Autodesk Inventor part; units mm, degrees
ref_plane "YZ Plane" through (0, 0, 0) normal (1, 0, 0) x (0, 1, 0)
ref_plane "XZ Plane" through (0, 0, 0) normal (0, 1, 0) x (-1, 0, 0)
ref_plane "XY Plane" through (0, 0, 0) normal (0, 0, 1) x (1, 0, 0)
sketch "スケッチ2" plane through (0, 0, 0) normal (0, 1, 0) x (-1, 0, 0)
  line L0 (43, -215) -> (-441.4, 962.3333)
  line L1 (32, 0) -> (32, -200)
  line L2 (0, 0) -> (0, -200)
  line L3 (32, 0) -> (0, 0)
  line L4 (16, 0) -> (16, -149.3765)
  line L5 (32, -200) -> (0, -200)
  dimension "d0" = 50.6234
ref_plane "作業平面1" through (-32, 0, -200) normal (0, 0, 1) x (1, 0, 0)
sketch "スケッチ5" plane through (-32, 0, -200) normal (0, 0, 1) x (1, 0, 0)
  line L0 (0, -16) -> (32, -16)
  line L1 (32, -16) -> (32, 16)
  line L2 (32, 16) -> (0, 16)
  line L3 (0, 16) -> (0, -16)
  line L4 (0, -16) -> (32, 16) construction
  line L5 (32, -16) -> (0, 16) construction
  line L6 (29.7, -13.7) -> (2.3, -13.7)
  line L7 (2.3, -13.7) -> (2.3, 13.7)
  line L8 (2.3, 13.7) -> (29.7, 13.7)
  line L9 (29.7, 13.7) -> (29.7, -13.7)
  point P0 (32, 0)
  point P1 (16, 0)
  dimension "d7" = 32
  dimension "d8" = 32
  dimension "d9" = 2.3
extrude "押し出し2" add sketch "スケッチ5" along normal blind 70
sketch "スケッチ6" plane through (-32, -16, -200) normal (0, -1, 0) x (1, 0, 0)
  line L0 (-11, -15) -> (473.4, 1162.3333)
  line L1 (16, 200) -> (16, 50.6235)
  point P0 (32, 200)
hole "穴1" at (-16, -16, -149.3765) direction (0, 1, 0) diameter 10 end through all
properties part number "ステア棒"
Read the model definition and answer for the solid it produces. Units are mm, in the model's axes. A direction names the side the tool comes from. Coordinates: 2 decimals unless noted, no trailing zeros. Write each loop counter-clockwise with the first axis right and the second up, starting at its lowest first coordinate (ties: lowest second). Pieces come first, ordered by that corner, then holes. Notation, with made-up numbers: (67.25, 41) - (75.25, 41) arc R27 ccw to (75.25, 73) - close; hole circle Ø5 at (10, 37.25). An arc over 180 degrees is marked (long way). One line per question, with ' | ' between items.
Q1. Find section B-B, the plane y = -3. Write down the section's boundary in (x, z), plus the area to 3 significant figures.
Result set:
outline: (-32, -200) - (-29.7, -200) - (-29.7, -130) - (-32, -130) - close; (-2.3, -200) - (0, -200) - (0, -130) - (-2.3, -130) - close | area: 322 mm^2
Q2. Find section A-A, the plane x = -6. Write down the section's boundary in (y, z), plus the area to 3 significant figures.
Result set:
outline: (-16, -200) - (-13.7, -200) - (-13.7, -130) - (-16, -130) - close; (13.7, -200) - (16, -200) - (16, -130) - (13.7, -130) - close | area: 322 mm^2
Q3. Find section C-C, the plane z = -141.5. Write down the section's boundary in (x, y), plus the area to 3 significant figures.
Result set:
outline: (-32, -16) - (0, -16) - (0, 16) - (-32, 16) - close; hole (-29.7, -13.7) - (-2.3, -13.7) - (-2.3, 13.7) - (-29.7, 13.7) - close | area: 273 mm^2
Q4. Determine the mould class of faces 3 (the cylindrical face through (-17.502, 14.866, -154.146)), 4 (the flat face through (-32, 0, -165)), 5 (the flat face through (-2, 0, -200)) for opening direction Z: +Z half, -Z half, draft (parallel to the pull), parting line (faces both ways), or undercut.
Result set:
face 3: undercut | face 4: draft | face 5: -Z half
Q5. Find section D-D, the plane x = -16. Write down the section's boundary in (y, z), plus the area to 3 significant figures.
Result set:
outline: (-16, -200) - (-13.7, -200) - (-13.7, -154.38) - (-16, -154.38) - close; (-16, -144.38) - (-13.7, -144.38) - (-13.7, -130) - (-16, -130) - close; (13.7, -200) - (16, -200) - (16, -154.38) - (13.7, -154.38) - close; (13.7, -144.38) - (16, -144.38) - (16, -130) - (13.7, -130) - close | area: 276 mm^2
Q6. Consider L1, parallel to Y at x = -26, z = -144; L2, parallel to X at y = 7, z = -196; L3, parallel to Z at x = -16, y = -15.1. Determine where each line is inside the solid, lowest interval first. Write a range as [from, to].
Result set:
L1: [-16, -13.7], [13.7, 16] | L2: [-32, -29.7], [-2.3, 0] | L3: [-200, -154.38], [-144.38, -130]
Q7. For faces 1 (the flat face through (-2.3, 0, -165)), 2 (the cylindrical face through (-17.502, -14.834, -154.146)), determine the directions among +Z, -Z, +X, -X, +Y, -Y from which every point of the face is accessible in a straight line to the end or side of a thin tool.
Result set:
face 1: +Z, -Z | face 2: +Y, -Y
